```python
from build123d import *

# Parameters (mm, degrees)
SKETCH1_W           = 12.7
SKETCH1_H           = 14.9987
SKETCH1_W_2         = 21.59
SKETCH1_H_2         = 36.5125
SKETCH3_R           = 3.3734375
CUT_EXTRUDE1_DEPTH  = 11.43
SKETCH5_R           = 4.7625
BOSS_EXTRUDE1_DEPTH = 6.35


with BuildPart() as part:
    # Sketch1 → Revolve1 (revolve)
    with BuildSketch(Plane(origin=(0, 0, 0), x_dir=(-1, 0, 0), z_dir=(0, 1, 0)), mode=Mode.PRIVATE) as revolve1_sk:
        Polygon((0, 0), (0, 46.99), (-20.32, 46.99), (-20.32, 36.5125), (-20.32, 0), align=None)
        Polygon((6.35, 73.550123262), (0, 73.550123262), (0, 46.99), (0, 0), (71.12, 0), (71.12, 14.9987), (71.12, 144.605660924), (58.245660924, 157.48), (19.224339076, 157.48), (6.35, 144.605660924), align=None)
        with Locations((77.47, 7.49935)):
            Rectangle(SKETCH1_W, SKETCH1_H)
        Polygon((83.82, 14.9987), (83.82, 0), (90.17, 0), (90.17, 24.13), (83.82, 24.13), align=None)
        with Locations((-31.115, 18.25625)):
            Rectangle(SKETCH1_W_2, SKETCH1_H_2)
    revolve(revolve1_sk.sketch.rotate(Axis((0, 0, 0), (-1, 0, 0)), 180), axis=Axis((0, 0, 0), (-1, 0, 0)))

    # Sketch3 → Cut-Extrude1 (cut)
    with BuildSketch(Plane(origin=(-71.12, 0, 0), x_dir=(0, -1, 0), z_dir=(-1, 0, 0))):
        with Locations(Location((-22.394618112, 30.823547486, 0), (0, 0, 90))):
            Circle(SKETCH3_R)
        with Locations(Location((22.394618112, 30.823547486, 0), (0, 0, 90))):
            Circle(SKETCH3_R)
        with Locations(Location((36.235253271, -11.773547486, 0), (0, 0, 90))):
            Circle(SKETCH3_R)
        with Locations(Location((0, -38.1, 0), (0, 0, 90))):
            Circle(SKETCH3_R)
        with Locations(Location((-36.235253271, -11.773547486, 0), (0, 0, 90))):
            Circle(SKETCH3_R)
    extrude(amount=-CUT_EXTRUDE1_DEPTH, mode=Mode.SUBTRACT)

    # Sketch5 → Boss-Extrude1 (add)
    with BuildSketch(Plane.YZ):
        with Locations(Location((28.956, 50.153263184, 0), (0, 0, 270))):
            Circle(SKETCH5_R)
        with Locations(Location((-28.956, 50.153263184, 0), (0, 0, 270))):
            Circle(SKETCH5_R)
        with Locations(Location((-57.912, 0, 0), (0, 0, 270))):
            Circle(SKETCH5_R)
        with Locations(Location((-28.956, -50.153263184, 0), (0, 0, 270))):
            Circle(SKETCH5_R)
        with Locations(Location((28.956, -50.153263184, 0), (0, 0, 270))):
            Circle(SKETCH5_R)
        with Locations(Location((57.912, 0, 0), (0, 0, 270))):
            Circle(SKETCH5_R)
    extrude(amount=BOSS_EXTRUDE1_DEPTH)


solid = part.part
```
Read the model definition and answer for the solid it produces. Units are mm, in the model's axes. A direction names the side the tool comes from. Give positions to 0.01 mm unless a question says otherwise; leave off trailing zeros. Order: outer loops, then holes, each group sorted by start corner. A loop starts at its lowest first (then second) coordinate and runs counter-clockwise, first axis right, second up. Notation, with made-up numbers: (72, -4) -> (87, -4) arc R13 cw to (87, 4) -> close; hole circle Ø11 at (-12, 68). An arc over 180 degrees is marked (long way). Write item = value, one per line.
1. Straight lines are drawn through the part: line 1 along X through (y, z) = (60.5, -98.5); line 2 along X through (y, z) = (13, 36); line 3 along Y through (x, z) = (29.5, 2.5). For each, find the intervals that lie inside material, in ascending order.
Numbers:
line_1 = -71.12 to -6.35
line_2 = -71.12 to 20.32
line_3 = -36.43 to 36.43
2. The mould has two halves that part along X. Classify faces 6 (the face through (-70.315, 141.953, 31.522)), 7 (the face through (-86.951, -7.248, -23.016)), 8 (the face through (41.91, -1, -1)), 9 (the face through (-83.82, 10.4, 11.1)): +X half, -X half, draft (parallel to the pull), parting line (faces both ways), or undercut.
Numbers:
face_6 = -X half
face_7 = draft
face_8 = +X half
face_9 = undercut
3. A cutting plane is placed at A-A, the plane x = 28. Write down the section's boundary in (y, z) (1 decimal), and give its area (3 significant figures).
Numbers:
outline = circle Ø73 at (0, 0)
area = 4,190 mm²
4. A cutting plane is placed at B-B, the plane x = -32. Write down the section's boundary in (y, z).
Numbers:
outline = circle Ø314.96 at (0, 0)
5. For faces 1 (the face through (6.35, -58, 0)), 2 (the face through (6.35, 29, -50)), 3 (the face through (6.35, -29, -50)), 4 (the face through (3.131, 30.387, -54.696)), 5 (the face through (-77.559, -0.659, 14.984)), determine the directions among +Z, -Z, +X, -X, +Y, -Y from which every point of the face is accessible in a straight line to the end or side of a thin tool.
Numbers:
face_1 = +Z, -Z, +X, -Y
face_2 = -Z, +X, +Y
face_3 = -Z, +X, -Y
face_4 = +X
face_5 = none
6. Given pin 1 (6 mm diameter, centred on x = -51, z = 118, fed in from +Y); pin 2 (7.5 mm diameter, centred on y = 27.5, z = -51, fed in from +X); pin 3 (10 mm diameter, centred on x = -29, y = -24, fed in from -Z), each flat-ended and moving along its own axis, determine where each tip first touches the part or whether it passes through.
Numbers:
pin_1 = 107.59
pin_2 = 6.35
pin_3 = -156.33
